from build123d import *

# Parameters (mm, degrees)
BOSS_EXTRUDE1_DEPTH = 23.333333333
F_20_0MM_1_D        = 20
SCALE_1_SCALE       = 0.3
EXTRUDE_1_DEPTH     = 7
SKETCH_3_R          = 0.9
CUT_EXTRUDE_1_DEPTH = 8
SKETCH_4_R          = 6
CUT_EXTRUDE_2_DEPTH = 8


with BuildPart() as part:
    # Sketch2 → Boss-Extrude1 (new body)
    with BuildSketch(Plane(origin=(0, 0, 0), x_dir=(1, 0, 0), z_dir=(0, 1, 0))):
        Polygon((-170, -90), (-50, -90), (-50, 90), (-170, 90), (-240, 40), (-240, -40), align=None)
    extrude(amount=BOSS_EXTRUDE1_DEPTH)

    # Ø20.0mm 맞춤핀 구멍1 (through all)
    with Locations(Plane(origin=(0, 23.333333333, 0), x_dir=(1, 0, 0), z_dir=(0, 1, 0))):
        with Locations((-204.389232105, 22.557395049), (-204.389232105, -22.557395049), (-112.996294866, 55), (-112.996294866, -55)):
            Hole(F_20_0MM_1_D / 2)


with BuildPart() as part_1:
    # 축척1: scaled about (-135.896414653, 11.666666667, 0)
    add(part.part.scale(SCALE_1_SCALE).moved(Location((-95.127490257, 8.166666667, 0))))

    # 스케치1 → 보스-돌출1 (add)
    with BuildSketch(Plane(origin=(0, 15.166666667, 0), x_dir=(1, 0, 0), z_dir=(0, 1, 0))):
        Polygon((-95.127490257, -7.5), (-100.127490257, -27), (-110.127490257, -27), (-110.127490257, 27), (-100.127490257, 27), (-95.127490257, 7.5), align=None)
    extrude(amount=-EXTRUDE_1_DEPTH)

    # 스케치3 → 컷-돌출1 (cut, through all)
    with BuildSketch(Plane.XZ.offset(-8.166666667)):
        with Locations((-97.627490257, 3.5)):
            Circle(SKETCH_3_R)
        with Locations((-97.627490257, -3.5)):
            Circle(SKETCH_3_R)
    extrude(amount=-CUT_EXTRUDE_1_DEPTH, mode=Mode.SUBTRACT)

    # 스케치4 → 컷-돌출2 (cut, through all)
    with BuildSketch(Plane.XZ.offset(-8.166666667)):
        with Locations((-129.026378717, -16.5)):
            Circle(SKETCH_4_R)
    extrude(amount=-CUT_EXTRUDE_2_DEPTH, mode=Mode.SUBTRACT)


solid = part_1.part
Model file for the job. Use its own axes, mm. Give positions to 0.01 mm unless a question says otherwise; leave off trailing zeros. Loops run counter-clockwise (first coordinate to the right, second up) from the corner with the lowest first, then second, coordinate; pieces in that order, holes last.
Item 1: Mould opens along X. For faces 1 (the face through (-156.77, 11.62, 19.4)), 2 (the face through (-98.527, 11.618, -3.46)), 3 (the face through (-123, 12, 27)), 4 (the face through (-158.06, 11.62, 4.24)) say: +X half, -X half, draft (parallel to the pull), parting line (faces both ways), or undercut.
Check values:
face 1: -X half
face 2: undercut
face 3: draft
face 4: undercut
Item 2: Slice it at C-C (z = 16.5). Write the cut outline in (x, y).
Check values:
outline: (-160.83, 8.17) - (-132.03, 8.17) - (-132.03, 15.17) - (-160.83, 15.17) - close; (-126.03, 8.17) - (-97.44, 8.17) - (-97.44, 15.17) - (-126.03, 15.17) - close
Item 3: Slice it at B-B (x = -128). Write the cut outline in (y, z).
Check values:
outline: (8.17, -27) - (15.17, -27) - (15.17, -22.41) - (8.17, -22.41) - close; (8.17, -10.59) - (15.17, -10.59) - (15.17, 13.68) - (8.17, 13.68) - close; (8.17, 19.32) - (15.17, 19.32) - (15.17, 27) - (8.17, 27) - close
Item 4: Drop flat-ended pins along their axis: P1, Ø5.5, axis at x = -156.44, z = 6.77, coming from the -Y side; P2, Ø4, axis at y = 11.5, z = 17.5, coming from the +X side. Give the stop position or say it passes through.
Check values:
P1: passes through
P2: stops at x = -97.18
Item 5: Slice it at A-A (z = -19). Write the cut outline in (x, y).
Check values:
outline: (-157.33, 8.17) - (-134.48, 8.17) - (-134.48, 15.17) - (-157.33, 15.17) - close; (-123.57, 8.17) - (-98.08, 8.17) - (-98.08, 15.17) - (-123.57, 15.17) - close
Item 6: Drill centre lines: line 1 along Z through (x, y) = (-129, 14.75); line 2 along Z through (x, y) = (-130, 10.25); line 3 along X through (y, z) = (10.5, -19.5). Where is each one in solid material? Low to high.
Check values:
line 1: z = -27 to -22.5, -10.5 to 13.5, 19.5 to 27
line 2: z = -27 to -22.42, -10.58 to 13.66, 19.34 to 27
line 3: x = -156.63 to -134.22, -123.83 to -98.2
